Drawing for the job (mm, zero at the part's lowest x, y, z). Round coordinates to 2 decimals unless told otherwise and drop trailing zeros. Write each loop counter-clockwise with the first axis right and the second up, starting at its lowest first coordinate (ties: lowest second). Pieces come first, ordered by that corner, then holes.
Item 1: Band-saw the part on C-C, the plane z = 4.75. Count the separate pieces of the cut face and the enclosed holes in it.
Item 2: Band-saw the part on A-A, the plane x = 19.05. Write the cut outline in (y, z).
Item 3: Wall check: probe 1 along Z at (x, y) = (28.5, 4.15); probe 2 along X at (y, z) = (1.9, 0.5); probe 3 along X at (y, z) = (0.75, 0.5) (1 decimal). Give the ranges that are in metal, low to high.
Item 4: Band-saw the part on B-B, the plane y = 1.7. Write the cut outline in (x, z) (1 decimal), then the cut area to 3 significant figures.
Item 5: Mould opens along Y. For the marked faces 1, 2, 3 and 4 say: +Y half, -Y half, draft (parallel to the pull), parting line (faces both ways), or undercut.
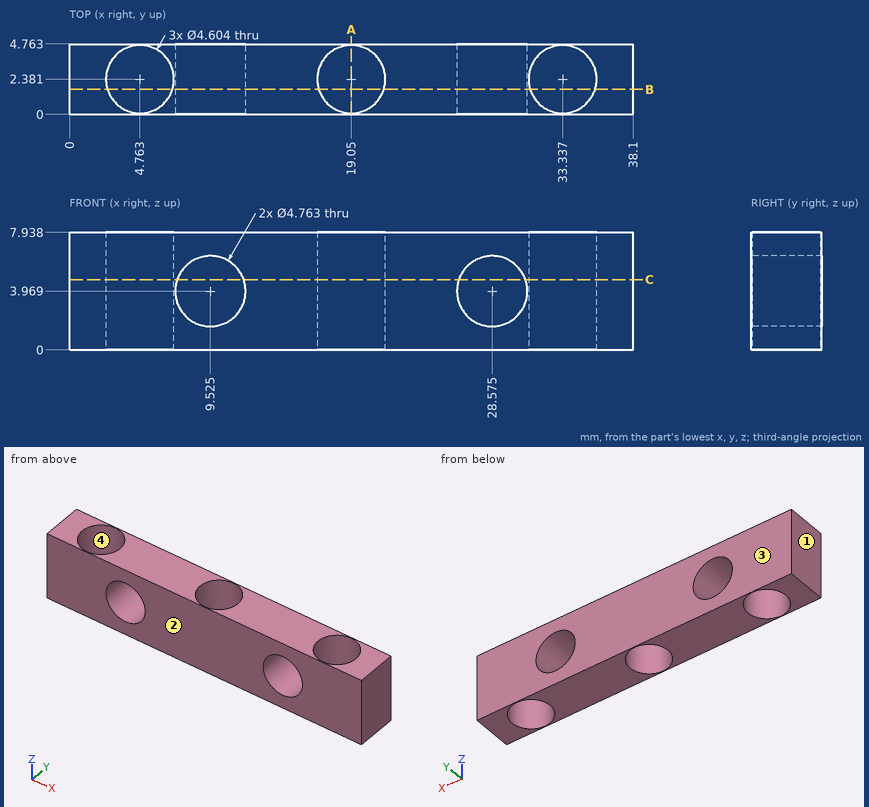
Results:
1. separate pieces: 3
1. enclosed holes: 3
2. outline: (0, 0) - (0.08, 0) - (0.08, 7.94) - (0, 7.94) - close; (4.68, 0) - (4.76, 0) - (4.76, 7.94) - (4.68, 7.94) - close
3. probe 1: z = 0 to 1.59, 6.35 to 7.94
3. probe 2: x = 0 to 2.51, 7.01 to 16.8, 21.3 to 31.09, 35.59 to 38.1
3. probe 3: x = 0 to 3.1, 6.4 to 17.4, 20.7 to 31.7, 35 to 38.1
4. outline: (0, 0) - (2.6, 0) - (2.6, 7.9) - (0, 7.9) - close; (7, 0) - (16.9, 0) - (16.9, 7.9) - (7, 7.9) - close; (21.2, 0) - (31.1, 0) - (31.1, 7.9) - (21.2, 7.9) - close; (35.5, 0) - (38.1, 0) - (38.1, 7.9) - (35.5, 7.9) - close; hole circle Ø4.8 at (9.5, 4); hole circle Ø4.8 at (28.6, 4)
4. area: 162 mm2
5. face 1: draft
5. face 2: -Y half
5. face 3: +Y half
5. face 4: undercut
